from build123d import *

# Parameters (mm, degrees)
SPUR_START             = 18.857514679
SPUR_GEAR_GB_OUTLINE_R = 1.5
SPUR_GEAR_GB_DEPTH     = 4
CUT_EXTRUDE_START      = -10
CUT_EXTRUDE_1_DEPTH    = 10
EXTRUDE_START          = -4
SKETCH_3_R             = 1.5
EXTRUDE_1_DEPTH        = 4
SKETCH_5_R             = 0.6
CUT_EXTRUDE_2_DEPTH    = 10


# Read off the part's stored shape, not the designer's step: spur gear_gb
with BuildPart() as part:
    # spur gear_gb outline → spur gear_gb (new body)
    with BuildSketch(Plane.YZ.offset(SPUR_START)):
        with BuildLine():
            ThreePointArc((-2.124081285, 2.218549628), (-2.409806694, 2.279250398), (-2.69701173, 2.332512579))
            ThreePointArc((-2.69701173, 2.332512579), (-3.581509704, 1.114965359), (-3.953511283, -0.34324338))
            ThreePointArc((-3.953511283, -0.34324338), (-4.604572817, -0.318084007), (-5.25563435, -0.34324338))
            ThreePointArc((-5.25563435, -0.34324338), (-5.627635929, 1.114965359), (-6.512133903, 2.332512579))
            ThreePointArc((-6.512133903, 2.332512579), (-6.799338939, 2.279250398), (-7.085064348, 2.218549628))
            ThreePointArc((-7.085064348, 2.218549628), (-7.436298774, 0.75519995), (-7.221951093, -0.734368099))
            ThreePointArc((-7.221951093, -0.734368099), (-7.833081593, -0.960274331), (-8.424955943, -1.232669023))
            ThreePointArc((-8.424955943, -1.232669023), (-9.326672913, -0.027818656), (-10.609777638, 0.75856558))
            ThreePointArc((-10.609777638, 0.75856558), (-10.854737938, 0.599449132), (-11.095484616, 0.434026553))
            ThreePointArc((-11.095484616, 0.434026553), (-10.859983236, -1.052343859), (-10.091918787, -2.346497986))
            ThreePointArc((-10.091918787, -2.346497986), (-10.570079176, -2.789077647), (-11.012658837, -3.267238036))
            ThreePointArc((-11.012658837, -3.267238036), (-12.306812964, -2.499173587), (-13.793183376, -2.263672207))
            ThreePointArc((-13.793183376, -2.263672207), (-13.958605955, -2.504418885), (-14.117722403, -2.749379185))
            ThreePointArc((-14.117722403, -2.749379185), (-13.331338167, -4.03248391), (-12.1264878, -4.93420088))
            ThreePointArc((-12.1264878, -4.93420088), (-12.398882492, -5.52607523), (-12.624788724, -6.13720573))
            ThreePointArc((-12.624788724, -6.13720573), (-14.114356773, -5.922858049), (-15.577706451, -6.274092475))
            ThreePointArc((-15.577706451, -6.274092475), (-15.638407221, -6.559817884), (-15.691669402, -6.84702292))
            ThreePointArc((-15.691669402, -6.84702292), (-14.474122182, -7.731520894), (-13.015913443, -8.103522473))
            ThreePointArc((-13.015913443, -8.103522473), (-13.041072816, -8.754584007), (-13.015913443, -9.40564554))
            ThreePointArc((-13.015913443, -9.40564554), (-14.474122182, -9.777647119), (-15.691669402, -10.662145093))
            ThreePointArc((-15.691669402, -10.662145093), (-15.638407221, -10.949350129), (-15.577706451, -11.235075538))
            ThreePointArc((-15.577706451, -11.235075538), (-14.114356773, -11.586309964), (-12.624788724, -11.371962283))
            ThreePointArc((-12.624788724, -11.371962283), (-12.398882492, -11.983092783), (-12.1264878, -12.574967133))
            ThreePointArc((-12.1264878, -12.574967133), (-13.331338167, -13.476684103), (-14.117722403, -14.759788828))
            ThreePointArc((-14.117722403, -14.759788828), (-13.958605955, -15.004749128), (-13.793183376, -15.245495806))
            ThreePointArc((-13.793183376, -15.245495806), (-12.306812964, -15.009994426), (-11.012658837, -14.241929977))
            ThreePointArc((-11.012658837, -14.241929977), (-10.570079176, -14.720090366), (-10.091918787, -15.162670027))
            ThreePointArc((-10.091918787, -15.162670027), (-10.859983236, -16.456824154), (-11.095484616, -17.943194566))
            ThreePointArc((-11.095484616, -17.943194566), (-10.854737938, -18.108617145), (-10.609777638, -18.267733593))
            ThreePointArc((-10.609777638, -18.267733593), (-9.326672913, -17.481349357), (-8.424955943, -16.27649899))
            ThreePointArc((-8.424955943, -16.27649899), (-7.833081594, -16.548893683), (-7.221951093, -16.774799914))
            ThreePointArc((-7.221951093, -16.774799914), (-7.436298774, -18.264367963), (-7.085064348, -19.727717641))
            ThreePointArc((-7.085064348, -19.727717641), (-6.799338939, -19.788418411), (-6.512133903, -19.841680592))
            ThreePointArc((-6.512133903, -19.841680592), (-5.627635929, -18.624133372), (-5.25563435, -17.165924633))
            ThreePointArc((-5.25563435, -17.165924633), (-4.604572817, -17.191084007), (-3.953511283, -17.165924633))
            ThreePointArc((-3.953511283, -17.165924633), (-3.581509704, -18.624133372), (-2.69701173, -19.841680592))
            ThreePointArc((-2.69701173, -19.841680592), (-2.409806694, -19.788418411), (-2.124081285, -19.727717641))
            ThreePointArc((-2.124081285, -19.727717641), (-1.772846859, -18.264367963), (-1.98719454, -16.774799914))
            ThreePointArc((-1.98719454, -16.774799914), (-1.376064039, -16.548893683), (-0.78418969, -16.27649899))
            ThreePointArc((-0.78418969, -16.27649899), (0.11752728, -17.481349357), (1.400632005, -18.267733593))
            ThreePointArc((1.400632005, -18.267733593), (1.645592305, -18.108617145), (1.886338983, -17.943194566))
            ThreePointArc((1.886338983, -17.943194566), (1.650837603, -16.456824154), (0.882773154, -15.162670027))
            ThreePointArc((0.882773154, -15.162670027), (1.360933543, -14.720090366), (1.803513204, -14.241929977))
            ThreePointArc((1.803513204, -14.241929977), (3.097667331, -15.009994426), (4.584037743, -15.245495806))
            ThreePointArc((4.584037743, -15.245495806), (4.749460322, -15.004749128), (4.90857677, -14.759788828))
            ThreePointArc((4.90857677, -14.759788828), (4.122192534, -13.476684103), (2.917342167, -12.574967133))
            ThreePointArc((2.917342167, -12.574967133), (3.18973686, -11.983092784), (3.415643091, -11.371962283))
            ThreePointArc((3.415643091, -11.371962283), (4.90521114, -11.586309964), (6.368560818, -11.235075538))
            ThreePointArc((6.368560818, -11.235075538), (6.429261588, -10.949350129), (6.482523769, -10.662145093))
            ThreePointArc((6.482523769, -10.662145093), (5.264976549, -9.777647119), (3.80676781, -9.40564554))
            ThreePointArc((3.80676781, -9.40564554), (3.831927184, -8.754584007), (3.80676781, -8.103522473))
            ThreePointArc((3.80676781, -8.103522473), (5.264976549, -7.731520894), (6.482523769, -6.84702292))
            ThreePointArc((6.482523769, -6.84702292), (6.429261588, -6.559817884), (6.368560818, -6.274092475))
            ThreePointArc((6.368560818, -6.274092475), (4.90521114, -5.922858049), (3.415643091, -6.13720573))
            ThreePointArc((3.415643091, -6.13720573), (3.18973686, -5.526075229), (2.917342167, -4.93420088))
            ThreePointArc((2.917342167, -4.93420088), (4.122192534, -4.03248391), (4.90857677, -2.749379185))
            ThreePointArc((4.90857677, -2.749379185), (4.749460322, -2.504418885), (4.584037743, -2.263672207))
            ThreePointArc((4.584037743, -2.263672207), (3.097667331, -2.499173587), (1.803513204, -3.267238036))
            ThreePointArc((1.803513204, -3.267238036), (1.360933543, -2.789077647), (0.882773154, -2.346497986))
            ThreePointArc((0.882773154, -2.346497986), (1.650837603, -1.052343859), (1.886338983, 0.434026553))
            ThreePointArc((1.886338983, 0.434026553), (1.645592305, 0.599449132), (1.400632005, 0.75856558))
            ThreePointArc((1.400632005, 0.75856558), (0.11752728, -0.027818656), (-0.78418969, -1.232669023))
            ThreePointArc((-0.78418969, -1.232669023), (-1.37606404, -0.960274331), (-1.98719454, -0.734368099))
            ThreePointArc((-1.98719454, -0.734368099), (-1.772846859, 0.75519995), (-2.124081285, 2.218549628))
        make_face()
        with Locations((-4.604572816, -8.754584007)):
            Circle(SPUR_GEAR_GB_OUTLINE_R, mode=Mode.SUBTRACT)
    extrude(amount=SPUR_GEAR_GB_DEPTH)

    # 草图2 → 切除-拉伸1 (cut)
    with BuildSketch(Plane(origin=(22.857514679, 0, 0), x_dir=(0, 0, -1), z_dir=(1, 0, 0)).offset(CUT_EXTRUDE_START)):
        with BuildLine():
            ThreePointArc((14.241929977, 1.803513204), (13.441652277, 2.410120568), (12.574967133, 2.917342167))
            ThreePointArc((12.574967133, 2.917342167), (13.476684103, 4.122192534), (14.759788828, 4.90857677))
            ThreePointArc((14.759788828, 4.90857677), (15.004749128, 4.749460322), (15.245495806, 4.584037743))
            ThreePointArc((15.245495806, 4.584037743), (15.009994426, 3.097667331), (14.241929977, 1.803513204))
        make_face()
        with BuildLine():
            ThreePointArc((11.371962283, 3.415643091), (11.586309964, 4.905211141), (11.235075538, 6.368560818))
            ThreePointArc((11.235075538, 6.368560818), (10.949350129, 6.429261588), (10.662145093, 6.482523769))
            ThreePointArc((10.662145093, 6.482523769), (9.777647119, 5.264976549), (9.40564554, 3.80676781))
            ThreePointArc((9.40564554, 3.80676781), (10.400463508, 3.669822202), (11.371962283, 3.415643091))
        make_face()
        with BuildLine():
            ThreePointArc((8.103522473, 3.80676781), (7.731520894, 5.264976549), (6.84702292, 6.482523769))
            ThreePointArc((6.84702292, 6.482523769), (6.559817884, 6.429261588), (6.274092475, 6.368560818))
            ThreePointArc((6.274092475, 6.368560818), (5.922858049, 4.905211141), (6.13720573, 3.415643091))
            ThreePointArc((6.13720573, 3.415643091), (7.108704505, 3.669822202), (8.103522473, 3.80676781))
        make_face()
        with BuildLine():
            ThreePointArc((4.93420088, 2.917342167), (4.03248391, 4.122192534), (2.749379185, 4.90857677))
            ThreePointArc((2.749379185, 4.90857677), (2.504418885, 4.749460322), (2.263672207, 4.584037743))
            ThreePointArc((2.263672207, 4.584037743), (2.499173587, 3.097667331), (3.267238036, 1.803513204))
            ThreePointArc((3.267238036, 1.803513204), (4.067515736, 2.410120568), (4.93420088, 2.917342167))
        make_face()
    extrude(amount=CUT_EXTRUDE_1_DEPTH, mode=Mode.SUBTRACT)

    # 草图3 → 凸台-拉伸1 (add)
    with BuildSketch(Plane(origin=(22.857514679, 0, 0), x_dir=(0, 0, -1), z_dir=(1, 0, 0)).offset(EXTRUDE_START)):
        with BuildLine():
            Line((2.323416592, 19.882976789), (4.7738451, -4.996641378))
            ThreePointArc((4.7738451, -4.996641378), (9.146652568, -8.585311723), (12.735322913, -4.212504255))
            Line((12.735322913, -4.212504255), (10.284894405, 20.667113912))
            ThreePointArc((10.284894405, 20.667113912), (5.912086937, 24.255784257), (2.323416592, 19.882976789))
        make_face()
        with Locations((6.304155498, 20.27504535)):
            Circle(SKETCH_3_R, mode=Mode.SUBTRACT)
        with Locations(Location((8.754584007, -4.604572816, 0), (0, 0, 180))):
            Circle(SKETCH_3_R, mode=Mode.SUBTRACT)
    extrude(amount=EXTRUDE_1_DEPTH)

    # 草图5 → 切除-拉伸2 (cut)
    with BuildSketch(Plane(origin=(22.857514679, 0, 0), x_dir=(0, 0, -1), z_dir=(1, 0, 0))):
        with Locations((8.109420565, 1.446128724)):
            Circle(SKETCH_5_R)
        with Locations((7.737682597, 5.429027561)):
            Circle(SKETCH_5_R)
    extrude(amount=-CUT_EXTRUDE_2_DEPTH, mode=Mode.SUBTRACT)


solid = part.part
Can you work these out from the model? Positions are in its coordinate system, mm. A direction names the side the tool comes from. Round coordinates to 2 decimals unless told otherwise and drop trailing zeros. Write each loop counter-clockwise with the first axis right and the second up, starting at its lowest first coordinate (ties: lowest second). Pieces come first, ordered by that corner, then holes. Notation, with made-up numbers: (-0.75, -38) -> (29.25, -38) arc R35 ccw to (29.25, -6) -> close; hole circle Ø6 at (-21.75, 7.5). An arc over 180 degrees is marked (long way). One line per question, with ' | ' between items. Start each with the question number.
1) Suppose I cut it at B-B on x = 21.7. Count the separate pieces of the cut face and the enclosed holes in it, then the cut area to 3 significant figures.
2) Suppose I cut it at C-C on y = 12. Write out the boundary of the cut face in (x, z), then the cut area to 3 significant figures.
3) I need wall thicknesses on line 1 (Z direction, x = 21.7, y = -4.5); line 2 (Y direction, x = 20.1, z = -18); line 3 (Y direction, x = 21.6, z = -4.75). Which ranges of each line are inside material? Lowest first, please. Write a range as [from, to].
4) On a 3-axis mill with a long thin cutter (end or side, diameter ignored), from which of +Z, -Z, +X, -X, +Y, -Y can I reach the whole of each face in a straight line? I mean faces 5 (the cylindrical face through (20.83, -7.437, -18.243)), 6 (the cylindrical face through (20.83, 0.133, -0.014)), 7 (the cylindrical face through (20.83, -3.59, -18.605)). Say none if no direction works.
5) Suppose I cut it at D-D on z = -15.75. Write out the boundary of the cut face in (x, y).
6) If we mould it in two halves opening along Y, with no side actions, what happens to faces 1 (the cylindrical face through (20.83, -1.774, -18.286)), 2 (the flat face through (22.858, 0, -9)), 3 (the cylindrical face through (20.89, 5.46, -7.14)), 4 (the cylindrical face through (20.83, -13.317, -13.461))? For each: released by +Y, released by -Y, zero draft, split by the parting line, or undercut.
7) Suppose I cut it at A-A on y = 19.5. Write out the boundary of the cut face in (x, z).
8) I'm going to push a flat-ended pin straight in: P1, Ø5, axis at y = 6, z = -14.5, coming from the -X side. Where does the tip first touch, or does it pass through?
Return value:
1) separate pieces: 1 | enclosed holes: 4 | area: 425 mm2
2) outline: (18.86, -11.14) -> (22.86, -11.14) -> (22.86, -3.1) -> (18.86, -3.1) -> close | area: 32.2 mm2
3) line 1: z = [-17.19, -10.25], [-7.26, -0.32] | line 2: y = [-11.01, -10.04], [-7.44, -5.4], [-3.81, -1.77], [0.83, 1.81] | line 3: y = [-12.46, 23.96]
4) face 5: +X, -X | face 6: +Z, +X, -X | face 7: -Z, +X, -X
5) outline: (18.86, -10.52) -> (22.86, -10.52) -> (22.86, 1.31) -> (18.86, 1.31) -> close
6) face 1: undercut | face 2: zero draft | face 3: undercut | face 4: released by -Y
7) outline: (18.86, -10.4) -> (22.86, -10.4) -> (22.86, -7.59) -> (18.86, -7.59) -> close; (18.86, -5.02) -> (22.86, -5.02) -> (22.86, -2.36) -> (18.86, -2.36) -> close
8) P1: passes through
